```python
from build123d import *

# Parameters (mm, degrees)
CROQUIS1_R              = 2.5
CROQUIS1_R_2            = 13.5
SALIENTE_EXTRUIR1_DEPTH = 4


with BuildPart() as part:
    # Croquis1 → Saliente-Extruir1 (new body)
    with BuildSketch(Plane(origin=(0, 0, 0), x_dir=(0, 0, -1), z_dir=(1, 0, 0))):
        with BuildLine():
            Line((-24, 3.5), (-24, -3.5))
            Line((-24, -3.5), (-12.081640676, -8.890104532))
            ThreePointArc((-12.081640676, -8.890104532), (0, -15), (12.081640676, -8.890104532))
            Line((12.081640676, -8.890104532), (24, -3.5))
            Line((24, -3.5), (24, 3.5))
            Line((24, 3.5), (11.269745357, 9.899133275))
            ThreePointArc((11.269745357, 9.899133275), (0, 15), (-11.269745357, 9.899133275))
            Line((-11.269745357, 9.899133275), (-24, 3.5))
        make_face()
        with Locations((-18.25, 0)):
            Circle(CROQUIS1_R, mode=Mode.SUBTRACT)
        with Locations((18.25, 0)):
            Circle(CROQUIS1_R, mode=Mode.SUBTRACT)
        Circle(CROQUIS1_R_2, mode=Mode.SUBTRACT)
    extrude(amount=SALIENTE_EXTRUIR1_DEPTH)


solid = part.part
```
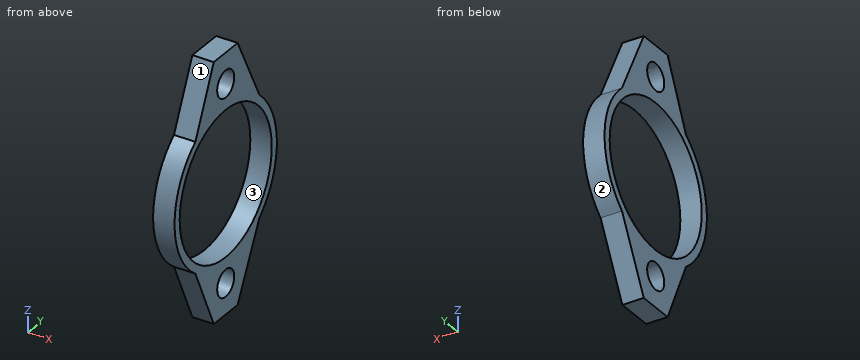
Geometry: final body of the model. Coordinates: model frame, mm. Face numbers are marked on the shaded views. Coordinates: 2 decimals unless noted, no trailing zeros. Order: outer loops, then holes, each group sorted by start corner. A loop starts at its lowest first (then second) coordinate and runs counter-clockwise, first axis right, second up. Notation, with made-up numbers: (-0.5, -2) -> (55.5, -2) arc R27 cw to (55.5, 17) -> close; hole circle Ø2 at (81.5, -17.75). An arc over 180 degrees is marked (long way). Write item = value, one per line.
(1) Cut plane D-D on y = 5. Return loops of the section in (x, z).
Solved:
outline = (0, -21.02) -> (4, -21.02) -> (4, -12.54) -> (0, -12.54) -> close; (0, 12.54) -> (4, 12.54) -> (4, 21.02) -> (0, 21.02) -> close
(2) Cut plane A-A on y = 0. Return loops of the section in (x, z).
Solved:
outline = (0, -24) -> (4, -24) -> (4, -20.75) -> (0, -20.75) -> close; (0, -15.75) -> (4, -15.75) -> (4, -13.5) -> (0, -13.5) -> close; (0, 13.5) -> (4, 13.5) -> (4, 15.75) -> (0, 15.75) -> close; (0, 20.75) -> (4, 20.75) -> (4, 24) -> (0, 24) -> close
(3) Cut plane B-B on x = 3.4. Return loops of the section in (y, z), plus the area to 3 significant figures.
Solved:
outline = (-8.89, -12.08) -> (-3.5, -24) -> (3.5, -24) -> (9.9, -11.27) arc R15 ccw to (9.9, 11.27) -> (3.5, 24) -> (-3.5, 24) -> (-8.89, 12.08) arc R15 ccw to start; hole circle Ø27 at (0, 0); hole circle Ø5 at (0, -18.25); hole circle Ø5 at (0, 18.25)
area = 327 mm²
(4) Cut plane C-C on z = -6. Return loops of the section in (x, y).
Solved:
outline = (0, -13.75) -> (4, -13.75) -> (4, -12.09) -> (0, -12.09) -> close; (0, 12.09) -> (4, 12.09) -> (4, 13.75) -> (0, 13.75) -> close
(5) Line query: line 1 (Y direction, x = 1.9, z = 0); line 2 (Z direction, x = 2.5, y = -2); line 3 (Y direction, x = 2.55, z = -3). Output: solid intervals per line, ascending.
Solved:
line_1 = -15 to -13.5, 13.5 to 15
line_2 = -24 to -19.75, -16.75 to -13.35, 13.35 to 16.75, 19.75 to 24
line_3 = -14.7 to -13.16, 13.16 to 14.7
(6) Pull-direction query (Z, two-part tool) for the marked faces 1, 2 and 3; classes: pulls with the +Z half, pulls with the -Z half, needs draft (parallel to the pull), parting line crosses it, or undercut.
Solved:
face_1 = pulls with the +Z half
face_2 = parting line crosses it
face_3 = undercut
(7) Pin query (flat end, axial travel): pin 1 Ø10 at (y, z) = (6.5, 8.5) entering from -X; pin 2 Ø1 at (y, z) = (11, 3) entering from +X; pin 3 Ø1.5 at (x, z) = (1.5, -13.5) entering from -Y; pin 4 Ø1.5 at (x, z) = (3, -15.5) entering from +Y. Return the tip coordinate at first contact, or that it passes through.
Solved:
pin_1 = 0
pin_2 = through
pin_3 = -8.59
pin_4 = 8.15
